The model under review builds one solid part; all positions refer to its coordinate system, in mm. A direction names the side the tool comes from. Coordinates: 2 decimals unless noted, no trailing zeros. Write each loop counter-clockwise with the first axis right and the second up, starting at its lowest first coordinate (ties: lowest second). Pieces come first, ordered by that corner, then holes.
```python
from build123d import *

# Parameters (mm, degrees)
F0_R     = 3.7382012242
F1_DEPTH = 3.556
F3_SCALE = 0.8
F4_R     = 1.27


with BuildPart() as f1:
    # F0 (on Front) → F1 (new body)
    with BuildSketch(Plane.XZ):
        with BuildLine():
            Line((-52.07, 181.6023319495), (-55.88, 181.6023319495))
            Line((-55.88, 181.6023319495), (-55.88, 86.1316665151))
            ThreePointArc((-55.88, 86.1316665151), (-52.0040063032, 75.6508869522), (-42.2413344101, 70.2139480257))
            ThreePointArc((-42.2413344101, 70.2139480257), (-14.9072200491, 47.7917837992), (-8.2826688201, 13.0639480257))
            ThreePointArc((-8.2826688201, 13.0639480257), (-14.8550807048, -4.3122984655), (0, -15.4683334849))
            ThreePointArc((0, -15.4683334849), (14.8550807048, -4.3122984655), (8.2826688201, 13.0639480257))
            ThreePointArc((8.2826688201, 13.0639480257), (14.9072200491, 47.7917837992), (42.2413344101, 70.2139480257))
            ThreePointArc((42.2413344101, 70.2139480257), (52.0040063032, 75.6508869522), (55.88, 86.1316665151))
            Line((55.88, 86.1316665151), (55.88, 181.6023319495))
            Line((55.88, 181.6023319495), (52.07, 181.6023319495))
            Line((52.07, 181.6023319495), (52.07, 105.4023319495))
            Line((52.07, 105.4023319495), (49.53, 105.4023319495))
            Line((49.53, 105.4023319495), (49.53, 181.6023319495))
            Line((49.53, 181.6023319495), (45.72, 181.6023319495))
            Line((45.72, 181.6023319495), (45.72, 105.4023319495))
            Line((45.72, 105.4023319495), (43.18, 105.4023319495))
            Line((43.18, 105.4023319495), (43.18, 181.6023319495))
            Line((43.18, 181.6023319495), (39.37, 181.6023319495))
            Line((39.37, 181.6023319495), (39.37, 105.4023319495))
            Line((39.37, 105.4023319495), (36.83, 105.4023319495))
            Line((36.83, 105.4023319495), (36.83, 181.6023319495))
            Line((36.83, 181.6023319495), (33.02, 181.6023319495))
            Line((33.02, 181.6023319495), (33.02, 105.4023319495))
            Line((33.02, 105.4023319495), (30.48, 105.4023319495))
            Line((30.48, 105.4023319495), (30.48, 181.6023319495))
            Line((30.48, 181.6023319495), (26.67, 181.6023319495))
            Line((26.67, 181.6023319495), (26.67, 105.4023319495))
            Line((26.67, 105.4023319495), (24.13, 105.4023319495))
            Line((24.13, 105.4023319495), (24.13, 181.6023319495))
            Line((24.13, 181.6023319495), (20.32, 181.6023319495))
            Line((20.32, 181.6023319495), (20.32, 105.4023319495))
            Line((20.32, 105.4023319495), (17.78, 105.4023319495))
            Line((17.78, 105.4023319495), (17.78, 181.6023319495))
            Line((17.78, 181.6023319495), (13.97, 181.6023319495))
            Line((13.97, 181.6023319495), (13.97, 105.4023319495))
            Line((13.97, 105.4023319495), (11.43, 105.4023319495))
            Line((11.43, 105.4023319495), (11.43, 181.6023319495))
            Line((11.43, 181.6023319495), (7.62, 181.6023319495))
            Line((7.62, 181.6023319495), (7.62, 105.4023319495))
            Line((7.62, 105.4023319495), (5.08, 105.4023319495))
            Line((5.08, 105.4023319495), (5.08, 181.6023319495))
            Line((5.08, 181.6023319495), (1.27, 181.6023319495))
            Line((1.27, 181.6023319495), (1.27, 105.4023319495))
            Line((1.27, 105.4023319495), (-1.27, 105.4023319495))
            Line((-1.27, 105.4023319495), (-1.27, 181.6023319495))
            Line((-1.27, 181.6023319495), (-5.08, 181.6023319495))
            Line((-5.08, 181.6023319495), (-5.08, 105.4023319495))
            Line((-5.08, 105.4023319495), (-7.62, 105.4023319495))
            Line((-7.62, 105.4023319495), (-7.62, 181.6023319495))
            Line((-7.62, 181.6023319495), (-11.43, 181.6023319495))
            Line((-11.43, 181.6023319495), (-11.43, 105.4023319495))
            Line((-11.43, 105.4023319495), (-13.97, 105.4023319495))
            Line((-13.97, 105.4023319495), (-13.97, 181.6023319495))
            Line((-13.97, 181.6023319495), (-17.78, 181.6023319495))
            Line((-17.78, 181.6023319495), (-17.78, 105.4023319495))
            Line((-17.78, 105.4023319495), (-20.32, 105.4023319495))
            Line((-20.32, 105.4023319495), (-20.32, 181.6023319495))
            Line((-20.32, 181.6023319495), (-24.13, 181.6023319495))
            Line((-24.13, 181.6023319495), (-24.13, 105.4023319495))
            Line((-24.13, 105.4023319495), (-26.67, 105.4023319495))
            Line((-26.67, 105.4023319495), (-26.67, 181.6023319495))
            Line((-26.67, 181.6023319495), (-30.48, 181.6023319495))
            Line((-30.48, 181.6023319495), (-30.48, 105.4023319495))
            Line((-30.48, 105.4023319495), (-33.02, 105.4023319495))
            Line((-33.02, 105.4023319495), (-33.02, 181.6023319495))
            Line((-33.02, 181.6023319495), (-36.83, 181.6023319495))
            Line((-36.83, 181.6023319495), (-36.83, 105.4023319495))
            Line((-36.83, 105.4023319495), (-39.37, 105.4023319495))
            Line((-39.37, 105.4023319495), (-39.37, 181.6023319495))
            Line((-39.37, 181.6023319495), (-43.18, 181.6023319495))
            Line((-43.18, 181.6023319495), (-43.18, 105.4023319495))
            Line((-43.18, 105.4023319495), (-45.72, 105.4023319495))
            Line((-45.72, 105.4023319495), (-45.72, 181.6023319495))
            Line((-45.72, 181.6023319495), (-49.53, 181.6023319495))
            Line((-49.53, 181.6023319495), (-49.53, 105.4023319495))
            Line((-49.53, 105.4023319495), (-52.07, 105.4023319495))
            Line((-52.07, 105.4023319495), (-52.07, 181.6023319495))
        make_face()
        Circle(F0_R, mode=Mode.SUBTRACT)
    extrude(amount=F1_DEPTH)


with BuildPart() as f1_1:
    # F3: moved
    add(f1.part.scale(F3_SCALE))

    # F4
    f4_edges = [f1_1.edges().sort_by_distance(p)[0] for p in [
        (33.02, 0, 145.281866),
        (31.496, -1.4224, 145.281866),
        (34.544, -1.4224, 145.281866),
        (39.624, -1.4224, 145.281866),
        (36.576, -1.4224, 145.281866),
        (38.1, 0, 145.281866),
        (38.1, -2.8448, 145.281866),
        (44.704, -1.4224, 145.281866),
        (41.656, -1.4224, 145.281866),
        (43.18, 0, 145.281866),
        (43.18, -2.8448, 145.281866),
        (29.464, -1.4224, 145.281866),
        (26.416, -1.4224, 145.281866),
        (27.94, 0, 145.281866),
        (27.94, -2.8448, 145.281866),
        (24.384, -1.4224, 145.281866),
        (21.336, -1.4224, 145.281866),
        (22.86, 0, 145.281866),
        (22.86, -2.8448, 145.281866),
        (19.304, -1.4224, 145.281866),
        (16.256, -1.4224, 145.281866),
        (17.78, 0, 145.281866),
        (17.78, -2.8448, 145.281866),
        (14.224, -1.4224, 145.281866),
        (11.176, -1.4224, 145.281866),
        (12.7, 0, 145.281866),
        (12.7, -2.8448, 145.281866),
        (9.144, -1.4224, 145.281866),
        (6.096, -1.4224, 145.281866),
        (7.62, 0, 145.281866),
        (7.62, -2.8448, 145.281866),
        (4.064, -1.4224, 145.281866),
        (1.016, -1.4224, 145.281866),
        (2.54, 0, 145.281866),
        (2.54, -2.8448, 145.281866),
        (-1.016, -1.4224, 145.281866),
        (-4.064, -1.4224, 145.281866),
        (-2.54, 0, 145.281866),
        (-2.54, -2.8448, 145.281866),
        (-6.096, -1.4224, 145.281866),
        (-9.144, -1.4224, 145.281866),
        (-7.62, 0, 145.281866),
        (-7.62, -2.8448, 145.281866),
        (-11.176, -1.4224, 145.281866),
        (-14.224, -1.4224, 145.281866),
        (-12.7, 0, 145.281866),
        (-12.7, -2.8448, 145.281866),
        (-16.256, -1.4224, 145.281866),
        (-19.304, -1.4224, 145.281866),
        (-17.78, 0, 145.281866),
        (-17.78, -2.8448, 145.281866),
        (-21.336, -1.4224, 145.281866),
        (-24.384, -1.4224, 145.281866),
        (-22.86, 0, 145.281866),
        (-22.86, -2.8448, 145.281866),
        (-26.416, -1.4224, 145.281866),
        (-29.464, -1.4224, 145.281866),
        (-27.94, 0, 145.281866),
        (-27.94, -2.8448, 145.281866),
        (-31.496, -1.4224, 145.281866),
        (-34.544, -1.4224, 145.281866),
        (-33.02, 0, 145.281866),
        (-33.02, -2.8448, 145.281866),
        (-36.576, -1.4224, 145.281866),
        (-39.624, -1.4224, 145.281866),
        (-38.1, 0, 145.281866),
        (-38.1, -2.8448, 145.281866),
        (-41.656, -1.4224, 145.281866),
        (-44.704, -1.4224, 145.281866),
        (-43.18, 0, 145.281866),
        (-43.18, -2.8448, 145.281866),
        (33.02, -2.8448, 145.281866),
    ]]
    fillet(f4_edges, radius=F4_R)


solid = f1_1.part
```
Item 1: Machinability: for faces 4 (the face through (-44.704, -1, 107)), 5 (the face through (-9.144, -1, 115)), which of the approach directions +Z, -Z, +X, -X, +Y, -Y give a long, thin tool a straight path to every point of the face, cutting with its end or side? Answer none if there is none.
Solved:
face 4: +Z, -Z, -X, +Y, -Y
face 5: +Z, +Y, -Y
Item 2: To check wall thickness, follow line 1 along Z through (x, y) = (0, -1.15); line 2 along Z through (x, y) = (9.5, -0.8); line 3 along X through (y, z) = (-2.2, 17.5). State the ranges of each line that lie inside material, in increasing order.
Solved:
line 1: z = -12.37 to -2.99, 2.99 to 84.32
line 2: z = -7.93 to 7.93, 33.48 to 84.32
line 3: x = -6.1 to 6.1
Item 3: Take a section at A-A, the plane z = 0. Write out the cut boundary in (x, y), plus the area to 3 significant figures.
Solved:
outline: (-12.37, -2.84) - (-2.99, -2.84) - (-2.99, 0) - (-12.37, 0) - close; (2.99, -2.84) - (12.37, -2.84) - (12.37, 0) - (2.99, 0) - close
area: 53.4 mm2
Item 4: For pin 1 (1.6 mm diameter, centred on x = 30.5, y = -1, fed in from +Z); pin 2 (1.6 mm diameter, centred on x = 36, y = -1.5, fed in from +Z), all flat-tipped, find the tip position at first contact; note any pin that passes through.
Solved:
pin 1: stops at z = 84.32
pin 2: stops at z = 144.73
Item 5: Mouldability with a two-part tool opening along X and no side actions: class faces 1 (the face through (-41.69, -1.4, 60.62)), 2 (the face through (-24.384, -1, 115)), 3 (the face through (44.704, -1, 106)) as pulls with the +X half, pulls with the -X half, needs draft (parallel to the pull), parting line crosses it, or undercut.
Solved:
face 1: pulls with the -X half
face 2: undercut
face 3: pulls with the +X half
